CAD build for the part. Positions are in the model's coordinates, mm. Face numbers are marked on the shaded views. A direction names the side the tool comes from. Coordinates: 2 decimals unless noted, no trailing zeros. Write each loop counter-clockwise with the first axis right and the second up, starting at its lowest first coordinate (ties: lowest second). Pieces come first, ordered by that corner, then holes. Notation, with made-up numbers: (17.5, -36) - (54.5, -36) arc R25 ccw to (54.5, -24) - close; hole circle Ø6 at (34, 12). An arc over 180 degrees is marked (long way). Answer in a Markdown table with one row per item. Add a question column.
Q1. Pin check, flat tips, straight feed: pin 1 (4 mm diameter, centred on y = -0.5, z = -3, fed in from +X); pin 2 (2 mm diameter, centred on y = 9.5, z = -2, fed in from +X); pin 3 (2 mm diameter, centred on y = 10.5, z = -7, fed in from -X). Stop position of each tip, or through.
Q2. Band-saw the part on B-B (y = 5.6). List the corners of the cut face in (x, z).
Q3. Band-saw the part on C-C (z = -8.25). List the corners of the cut face in (x, y).
Q4. Two-plate mould, pull along X, no slides. Class the marked faces 1, 2, 3 and 4: +X half, -X half, draft (parallel to the pull), parting line (faces both ways), or undercut.
Q5. Drill centre lines: line 1 along X through (y, z) = (5.25, -1.5); line 2 along X through (y, z) = (9.75, -4.5); line 3 along Y through (x, z) = (-6.75, -6). Where is each one in solid material? Low to high. Write a range as from..to.
Q6. Band-saw the part on A-A (x = -3.45). List the corners of the cut face in (y, z), and give its area (3 significant figures).
Q7. 3-axis set-ups, long thin cutter, end or side, ignore diameter. For the marked faces 5 and 6: which of +Z, -Z, +X, -X, +Y, -Y reach the whole face in a straight line?
Q8. Band-saw the part on D-D (x = -9.25). List the corners of the cut face in (y, z), and give its area (3 significant figures).
Autodesk Inventor part; units mm, degrees
ref_plane "YZ Plane" through (0, 0, 0) normal (1, 0, 0) x (0, 1, 0)
ref_plane "XZ Plane" through (0, 0, 0) normal (0, 1, 0) x (-1, 0, 0)
ref_plane "XY Plane" through (0, 0, 0) normal (0, 0, 1) x (1, 0, 0)
sketch "Sketch1" plane through (0, 0, 0) normal (0, 0, 1) x (1, 0, 0)
  line L0 (0, 0.5) -> (0, 9.6)
  arc A0 (0, 9.6) -> (-0.5, 10.1) centre (-0.5, 9.6) ccw
  line L1 (-0.5, 10.1) -> (-6.4, 10.1)
  arc A1 (-6.4, 10.1) -> (-6.9, 9.6) centre (-6.4, 9.6) ccw
  line L2 (-6.9, 9.6) -> (-6.9, 0.5)
  arc A2 (-6.9, 0.5) -> (-6.4, 0) centre (-6.4, 0.5) ccw
  line L3 (-6.4, 0) -> (-0.5, 0)
  arc A3 (-0.5, 0) -> (0, 0.5) centre (-0.5, 0.5) ccw
  line L4 (-2.6, 8.25) -> (-2.6, 8.8)
  line L5 (-1.15, 8.25) -> (-2.6, 8.25)
  line L6 (-1.15, 3.65) -> (-1.15, 8.25)
  line L7 (-1.8, 3.65) -> (-1.15, 3.65)
  line L8 (-1.8, 2.85) -> (-1.8, 3.65)
  line L9 (-1.15, 2.85) -> (-1.8, 2.85)
  line L10 (-1.15, 1.75) -> (-1.15, 2.85)
  line L11 (-2.15, 1.75) -> (-1.15, 1.75)
  line L12 (-2.15, 0.75) -> (-2.15, 1.75)
  line L13 (-4.75, 0.75) -> (-2.15, 0.75)
  line L14 (-4.75, 1.75) -> (-4.75, 0.75)
  line L15 (-5.75, 1.75) -> (-4.75, 1.75)
  line L16 (-5.75, 2.85) -> (-5.75, 1.75)
  line L17 (-5.1, 2.85) -> (-5.75, 2.85)
  line L18 (-5.1, 3.65) -> (-5.1, 2.85)
  line L19 (-5.75, 3.65) -> (-5.1, 3.65)
  line L20 (-5.75, 8.25) -> (-5.75, 3.65)
  line L21 (-4.3, 8.25) -> (-5.75, 8.25)
  line L22 (-4.3, 8.8) -> (-4.3, 8.25)
  line L23 (-2.6, 8.8) -> (-4.3, 8.8)
  circle A4 centre (-3.45, 5.6) radius 0.9
  circle A5 centre (-3.45, 5.6) radius 11.4128
  line L24 (-7.1, 0.5) -> (-7.1, 9.6)
  arc A6 (-6.4, 10.3) -> (-7.1, 9.6) centre (-6.4, 9.6) ccw
  line L25 (-6.4, 10.3) -> (-0.5, 10.3)
  arc A7 (0.2, 9.6) -> (-0.5, 10.3) centre (-0.5, 9.6) ccw
  line L26 (0.2, 9.6) -> (0.2, 0.5)
  arc A8 (-0.5, -0.2) -> (0.2, 0.5) centre (-0.5, 0.5) ccw
  line L27 (-0.5, -0.2) -> (-6.4, -0.2)
  arc A9 (-7.1, 0.5) -> (-6.4, -0.2) centre (-6.4, 0.5) ccw
  point P0 (0, 0)
  dimension "d0" = 0.2
extrude "Extrusion1" add sketch "Sketch1" against normal blind 10 contours A5
properties part number "00_SM05LC-toRMS"
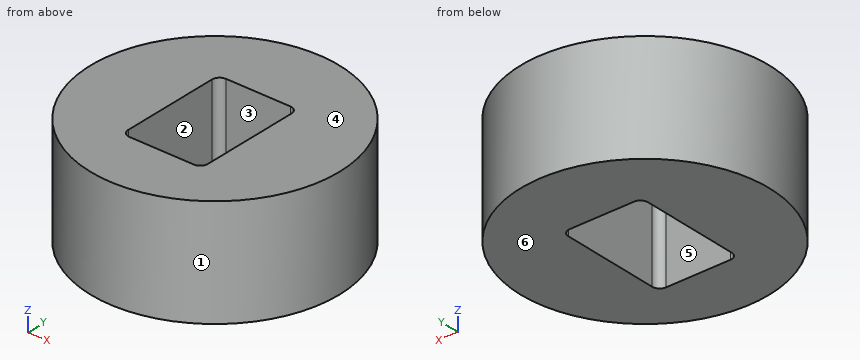
Checked values:
| question | item | result |
|---|---|---|
| 1 | pin 1 | stops at x = 7.2 |
| 1 | pin 2 | stops at x = 7.59 |
| 1 | pin 3 | stops at x = -14.18 |
| 2 | outline | (-14.86, -10) - (-7.1, -10) - (-7.1, 0) - (-14.86, 0) - close; (0.2, -10) - (7.96, -10) - (7.96, 0) - (0.2, 0) - close |
| 3 | outline | circle Ø22.83 at (-3.45, 5.6); hole (-7.1, 0.5) arc R0.7 ccw to (-6.4, -0.2) - (-0.5, -0.2) arc R0.7 ccw to (0.2, 0.5) - (0.2, 9.6) arc R0.7 ccw to (-0.5, 10.3) - (-6.4, 10.3) arc R0.7 ccw to (-7.1, 9.6) - close |
| 4 | face 1 | parting line |
| 4 | face 2 | undercut |
| 4 | face 3 | undercut |
| 4 | face 4 | draft |
| 5 | line 1 | x = -14.86..-7.1, 0.2..7.96 |
| 5 | line 2 | x = -14.08..-7.08, 0.18..7.18 |
| 5 | line 3 | y = -5.33..-0.11, 10.21..16.53 |
| 6 | outline | (-5.81, -10) - (-0.2, -10) - (-0.2, 0) - (-5.81, 0) - close; (10.3, -10) - (17.01, -10) - (17.01, 0) - (10.3, 0) - close |
| 6 | area | 123 mm² |
| 7 | face 5 | +Z, -Z |
| 7 | face 6 | -Z, +X, -X, +Y, -Y |
| 8 | outline | (-4.23, -10) - (15.43, -10) - (15.43, 0) - (-4.23, 0) - close |
| 8 | area | 197 mm² |
